Geometry: final body of the model. Coordinates: model frame, mm. A direction names the side the tool comes from. Round coordinates to 2 decimals unless told otherwise and drop trailing zeros. Loops run counter-clockwise (first coordinate to the right, second up) from the corner with the lowest first, then second, coordinate; pieces in that order, holes last. Notation, with made-up numbers: (8, -35.75) - (28, -35.75) arc R10 ccw to (28, -27.75) - close; hole circle Ø2 at (-3.75, -36.75). An arc over 180 degrees is marked (long way). Answer as a JSON object with one key per item and string values. Group by question number.
Item 1: Section C-C (z = 0.8). Return the cut outline in (x, y), plus the area to 3 significant figures.
Item 2: Line query: line 1 (Y direction, x = 0, z = 3.35); line 2 (Z direction, x = -2.25, y = 3); line 3 (Y direction, x = 2.25, z = 3.3). Output: solid intervals per line, ascending.
Item 3: Reachability of faces 1 (the face through (-1.65, 7.44, 1.25)), 2 (the face through (7, -2, 2.54)) from +Z, -Z, +X, -X, +Y, -Y: full face, straight path, thin tool, end or side. Return the list, or none.
Item 4: Section D-D (z = 3.8). Return the cut outline in (x, y) (1 decimal), plus the area to 3 significant figures.
Item 5: Section A-A (x = 0). Return the cut outline in (y, z).
Item 6: First-contact query: pin 1 (7.5 mm diameter, centred on x = 1.5, y = -1, fed in from +Z); pin 2 (2 mm diameter, centred on y = 3.5, z = 1, fed in from +X); pin 3 (1 mm diameter, centred on x = 3.5, z = 3.5, fed in from -Y). Flat tips, straight axial feed; report the tip coordinate or a pass-through.
Autodesk Inventor part; units mm, degrees
ref_plane "YZ Plane" through (0, 0, 0) normal (1, 0, 0) x (0, 1, 0)
ref_plane "XZ Plane" through (0, 0, 0) normal (0, 1, 0) x (-1, 0, 0)
ref_plane "XY Plane" through (0, 0, 0) normal (0, 0, 1) x (1, 0, 0)
sketch "Sketch1" plane through (0, 0, 0) normal (0, 0, 1) x (1, 0, 0)
  circle A0 centre (0, 0) radius 7.62
  dimension "d0" = 15.24
extrude "Extrusion1" add sketch "Sketch1" along normal blind 2.54
sketch "Sketch2" plane through (0, 0, 2.54) normal (0, 0, 1) x (1, 0, 0)
  circle A0 centre (0, 0) radius 7.62
  circle A1 centre (0, 0) radius 7.0104
  dimension "d3" = 14.0208
extrude "Extrusion2" add sketch "Sketch2" along normal blind 2.54 contours A1
thread "Thread1"
sketch "Sketch3" plane through (0, 0, 5.08) normal (0, 0, 1) x (1, 0, 0)
  circle A0 centre (0, 0) radius 7.0104
  circle A1 centre (0, 0) radius 5.3975
  dimension "d8" = 10.795
extrude "Extrusion3" cut sketch "Sketch3" against normal blind 2.54 contours A1
properties part number "cap_a"
Values:
{
 "1": {"outline": "circle Ø15.24 at (0, 0)", "area": "182 mm^2"},
 "2": {"line 1": "y = -7.01 to -5.4, 5.4 to 7.01", "line 2": "z = 0 to 2.54", "line 3": "y = -6.64 to -4.91, 4.91 to 6.64"},
 "3": {"face 1": "+Z, -Z", "face 2": "+Z"},
 "4": {"outline": "circle Ø14 at (0, 0); hole circle Ø10.8 at (0, 0)", "area": "62.9 mm^2"},
 "5": {"outline": "(-7.62, 0) - (7.62, 0) - (7.62, 2.54) - (7.01, 2.54) - (7.01, 5.08) - (5.4, 5.08) - (5.4, 2.54) - (-5.4, 2.54) - (-5.4, 5.08) - (-7.01, 5.08) - (-7.01, 2.54) - (-7.62, 2.54) - close"},
 "6": {"pin 1": "stops at z = 5.08", "pin 2": "stops at x = 7.2", "pin 3": "stops at y = -6.34"}
}
